Model file for the job. Use its own axes, mm. A direction names the side the tool comes from. Give positions to 0.01 mm unless a question says otherwise; leave off trailing zeros. Loops run counter-clockwise (first coordinate to the right, second up) from the corner with the lowest first, then second, coordinate; pieces in that order, holes last. Notation, with made-up numbers: (38, -9.5) - (75, -9.5) arc R14 cw to (75, 15.5) - close; hole circle Ø3 at (52.25, 43.25). An arc over 180 degrees is marked (long way). Answer as CSV lines item,"result". Start each with the question number.
Item 1: Saw through at B-B on x = 0. Give the cut face in (y, z), plus the area to 3 significant figures.
Item 2: Saw through at C-C on y = -16.5. Give the cut face in (x, z).
Item 3: Saw through at D-D on x = 18. Give the cut face in (y, z).
Item 4: Drill centre lines: L1, parallel to Z at x = 0, y = -9; L2, parallel to Y at x = -5, z = 12.5 (3 decimals); L3, parallel to X at y = 5, z = 16.5 (3 decimals). Where is each one in solid material? Low to high. Write a range as from..to.
Item 5: Pull direction Z, two halves, no side cores. Call faces 1 (the cylindrical face through (4.77, -10.11, 8.7)), 2 (the cylindrical face through (2.307, 10.024, 2.766)), 3 (the flat face through (-0.4, 8.2, -20)), 4 (the flat face through (18, -22.5, 0)): pulls with the +Z half, pulls with the -Z half, needs draft (parallel to the pull), parting line crosses it, or undercut.
Item 6: Tool access for faces 5 (the cylindrical face through (-23, -17, 0)), 6 (the flat face through (-18, -22.5, 0)): list every direction of +Z, -Z, +X, -X, +Y, -Y with a clear straight run to the whole face (end or side of a thin tool).
Item 7: Saw through at A-A on z = 0. Give the cut face in (x, y), plus the area to 3 significant figures.
Item 8: Pin check, flat tips, straight feed: pin 1 (11.5 mm diameter, centred on x = 0, z = 7.2, fed in from -Y); pin 2 (4 mm diameter, centred on x = -20.5, y = -16.5, fed in from +Z). Stop position of each tip, or through.
from build123d import *

# Parameters (mm, degrees)
F0_W     = 60
F0_H     = 40
F1_DEPTH = 12.5
F2_R     = 8
F3_DEPTH = 40.001
F4_R     = 5
F5_DEPTH = 10
F6_R     = 5
F7_DEPTH = 25


with BuildPart() as f1:
    # F0 (on Front) → F1 (new body, symmetric)
    with BuildSketch(Plane.XZ):
        Rectangle(F0_W, F0_H)
    extrude(amount=F1_DEPTH, both=True)

    # F2 (on face) → F3 (cut, through all)
    with BuildSketch(Plane.XY.offset(20)):
        Circle(F2_R)
    extrude(amount=-F3_DEPTH, mode=Mode.SUBTRACT)

    # F4 (on face) → F5 (join)
    with BuildSketch(Plane.XZ.offset(12.5)):
        with Locations((-18, 0)):
            Circle(F4_R)
        with Locations((18, 0)):
            Circle(F4_R)
    extrude(amount=F5_DEPTH)

    # F6 (on face) → F7 (cut)
    with BuildSketch(Plane.XZ.offset(12.5)):
        with Locations((0, 7.201633)):
            Circle(F6_R)
    extrude(amount=-F7_DEPTH, mode=Mode.SUBTRACT)


solid = f1.part
Responses:
1,outline,"(-12.5, -20) - (-8, -20) - (-8, 2.2) - (-12.5, 2.2) - close; (-12.5, 12.2) - (-8, 12.2) - (-8, 20) - (-12.5, 20) - close; (8, -20) - (12.5, -20) - (12.5, 2.2) - (8, 2.2) - close; (8, 12.2) - (12.5, 12.2) - (12.5, 20) - (8, 20) - close"
1,area,"270 mm2"
2,outline,"circle Ø10 at (-18, 0); circle Ø10 at (18, 0)"
3,outline,"(-22.5, -5) - (-12.5, -5) - (-12.5, -20) - (12.5, -20) - (12.5, 20) - (-12.5, 20) - (-12.5, 5) - (-22.5, 5) - close"
4,L1,"-20..2.2, 12.2..20"
4,L2,"-12.5..-6.245, 6.245..12.5"
4,L3,"-30..-6.245, 6.245..30"
5,face 1,"undercut"
5,face 2,"undercut"
5,face 3,"pulls with the -Z half"
5,face 4,"needs draft"
6,face 5,"-Y"
6,face 6,"+Z, -Z, +X, -X, -Y"
7,outline,"(-30, -12.5) - (-23, -12.5) - (-23, -22.5) - (-13, -22.5) - (-13, -12.5) - (13, -12.5) - (13, -22.5) - (23, -22.5) - (23, -12.5) - (30, -12.5) - (30, 12.5) - (-30, 12.5) - close; hole circle Ø16 at (0, 0)"
7,area,"1,500 mm2"
8,pin 1,"y = -12.5"
8,pin 2,"z = 4.97"
